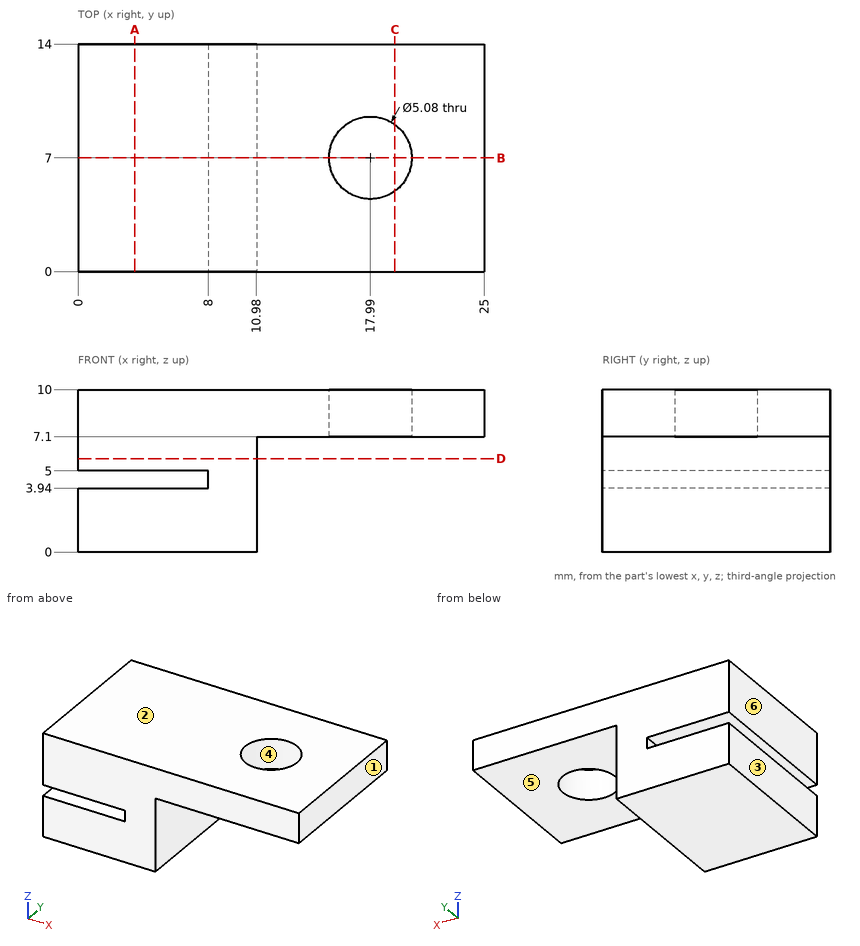
Could you check a few things on this drawing? It's one solid part, dimensions in mm from its lowest x, y, z. A direction names the side the tool comes from. Coordinates: 2 decimals unless noted, no trailing zeros. Order: outer loops, then holes, each group sorted by start corner. A loop starts at its lowest first (then second) coordinate and runs counter-clockwise, first axis right, second up.
1. I need wall thicknesses on line 1 (Z direction, x = 2, y = 5); line 2 (Y direction, x = 18, z = 7.75); line 3 (X direction, y = 6, z = 1.5). Which ranges of each line are inside material? Lowest first, please.
2. If we section it at D-D (z = 5.75): Please give me the cut outline in (x, y).
3. If we section it at B-B (y = 7): Please give me the cut outline in (x, z), then the cut area to 3 significant figures.
4. Thinking about a two-plate mould opening in X: for the marked faces 1, 2, 3 and 4, which applies, +X half, -X half, draft (parallel to the pull), parting line (faces both ways), or undercut?
5. I'm going to push flat-ended pins straight in: pin 1 (4 mm diameter, centred on y = 12.5, z = 3.5, fed in from +X); pin 2 (6.5 mm diameter, centred on x = 17.99, y = 7, fed in from -Z); pin 3 (0.8 mm diameter, centred on y = 6, z = 4.5, fed in from -X). Where does each tip first touch, or does it pass through?
6. If we section it at C-C (x = 19.5): Please give me the cut outline in (y, z).
7. If we section it at A-A (x = 3.5): Please give me the cut outline in (y, z), then the cut area to 3 significant figures.
8. For the marked faces 5 and 6, which set-ups out of +Z, -Z, +X, -X, +Y, -Y let a thin tool reach every point of the face, with its end or its side?
Entries:
1. line 1: z = 0 to 3.94, 5 to 10
1. line 2: y = 0 to 4.46, 9.54 to 14
1. line 3: x = 0 to 10.98
2. outline: (0, 0) - (10.98, 0) - (10.98, 14) - (0, 14) - close
3. outline: (0, 0) - (10.98, 0) - (10.98, 7.1) - (15.45, 7.1) - (15.45, 10) - (0, 10) - (0, 5) - (8, 5) - (8, 3.94) - (0, 3.94) - close; (20.53, 7.1) - (25, 7.1) - (25, 10) - (20.53, 10) - close
3. area: 127 mm2
4. face 1: +X half
4. face 2: draft
4. face 3: -X half
4. face 4: undercut
5. pin 1: stops at x = 10.98
5. pin 2: stops at z = 7.1
5. pin 3: stops at x = 8
6. outline: (0, 7.1) - (4.96, 7.1) - (4.96, 10) - (0, 10) - close; (9.04, 7.1) - (14, 7.1) - (14, 10) - (9.04, 10) - close
7. outline: (0, 0) - (14, 0) - (14, 3.94) - (0, 3.94) - close; (0, 5) - (14, 5) - (14, 10) - (0, 10) - close
7. area: 125 mm2
8. face 5: -Z, +X, +Y, -Y
8. face 6: +Z, -Z, -X, +Y, -Y
